from build123d import *

# Parameters (mm, degrees)
F1_DEPTH = 3.556
F3_DEPTH = 4.572
F4_R     = 9.984236
F5_DEPTH = 25.4


with BuildPart() as f1:
    # F0 (on Right) → F1 (new body)
    with BuildSketch(Plane.YZ):
        Polygon((44.500802, -31.851601), (44.500802, 64.160399), (-10.668, 64.160399), (-19.812001, 15.0876), (-53.340003, 4.7244), (-53.340003, -31.851601), align=None)
    extrude(amount=F1_DEPTH)

    # F2 (on face) → F3 (join)
    with BuildSketch(Plane.YZ.offset(3.556)):
        Polygon((-10.668, 64.160399), (-19.812001, 15.0876), (-53.340003, 4.7244), (-53.340003, -31.851601), (44.500802, -31.851601), (44.500802, 64.160399), align=None)
        Polygon((-8.029966, 60.985399), (41.325802, 60.985399), (41.325802, -28.676601), (-50.165003, -28.676601), (-50.165003, 2.382557), (-17.042049, 12.620561), align=None, mode=Mode.SUBTRACT)
    extrude(amount=F3_DEPTH)

    # F4 (on face) → F5 (cut)
    with BuildSketch(Plane(origin=(0, 0, 0), x_dir=(0, -1, 0), z_dir=(-1, 0, 0))):
        with Locations((-24.9936, 12.0396)):
            Circle(F4_R)
    extrude(amount=-F5_DEPTH, mode=Mode.SUBTRACT)


solid = f1.part
Model file for the job. Use its own axes, mm. A direction names the side the tool comes from. Give positions to 0.01 mm unless a question says otherwise; leave off trailing zeros. Order: outer loops, then holes, each group sorted by start corner. A loop starts at its lowest first (then second) coordinate and runs counter-clockwise, first axis right, second up. Notation, with made-up numbers: (54.5, 31) - (61.5, 31) arc R16 ccw to (61.5, 41) - close; hole circle Ø8 at (-22, -40). An arc over 180 degrees is marked (long way). Write item = value, one per line. Start each with the question number.
1. Probe line 1 along Y through (x, z) = (7.75, -19.5) (3 decimals); line 2 along Z through (x, y) = (6.75, 19); line 3 along X through (y, z) = (-14, 14). List the from-to ranges inside material, lowest first.
2. Drop flat-ended pins along their axis: P1, Ø4, axis at x = 1.5, y = -42, coming from the +Z side; P2, Ø23, axis at y = 24.99, z = 12.04, coming from the -X side. Give the stop position or say it passes through.
3. Cut at C-C, the plane z = 20. List the corners of the cut face in (x, y).
4. Cut at D-D, the plane y = -2.5. List the corners of the cut face in (x, z), and give its area (3 significant figures).
5. Two-plate mould, pull along Z, no slides. Class faces 1 (the flat face through (6, 41.326, 17)), 2 (the flat face through (4, -5, -31.852)), 3 (the flat face through (4, 17, 64.16)): pulls with the +Z half, pulls with the -Z half, needs draft (parallel to the pull), parting line crosses it, or undercut.
6. Which spindle directions (+Z, -Z, +X, -X, +Y, -Y) get a long thin tool onto all of the face, cutting with end or side? Do faces 4 (the flat face through (5.81, -33.84, 7.43)), 5 (the flat face through (0, 6, 6)). Say none if no direction does.
7. Cut at B-B, the plane z = -6.5. List the corners of the cut face in (x, y) (3 decimals), and give its area (3 significant figures).
8. Cut at A-A, the plane x = 5.5. List the corners of the cut face in (y, z) (3 decimals), and give its area (3 significant figures).
Taken from the geometry:
q1.line_1 = -53.34 to -50.165, 41.326 to 44.501
q1.line_2 = -31.85 to -28.68, 60.99 to 64.16
q1.line_3 = 0 to 3.56
q2.P1 = 8.85
q2.P2 = 0
q3.outline = (0, -18.9) - (8.13, -18.9) - (8.13, -15.67) - (3.56, -15.67) - (3.56, 18.97) - (0, 18.97) - close; (0, 31.02) - (3.56, 31.02) - (3.56, 41.33) - (8.13, 41.33) - (8.13, 44.5) - (0, 44.5) - close
q4.outline = (0, -31.85) - (8.13, -31.85) - (8.13, -28.68) - (3.56, -28.68) - (3.56, 60.99) - (8.13, 60.99) - (8.13, 64.16) - (0, 64.16) - close
q4.area = 370 mm²
q5.face_1 = undercut
q5.face_2 = pulls with the -Z half
q5.face_3 = pulls with the +Z half
q6.face_4 = +X
q6.face_5 = +Z, -Z, -X, +Y, -Y
q7.outline = (0, -53.34) - (8.128, -53.34) - (8.128, -50.165) - (3.556, -50.165) - (3.556, 41.326) - (8.128, 41.326) - (8.128, 44.501) - (0, 44.501) - close
q7.area = 377 mm²
q8.outline = (-53.34, -31.852) - (44.501, -31.852) - (44.501, 64.16) - (-10.668, 64.16) - (-19.812, 15.088) - (-53.34, 4.724) - close; hole (-50.165, -28.677) - (41.326, -28.677) - (41.326, 60.985) - (-8.03, 60.985) - (-17.042, 12.621) - (-50.165, 2.383) - close
q8.area = 1,140 mm²
